from build123d import *

# Parameters (mm, degrees)
SKETCH_1_W          = 180
SKETCH_1_H          = 128
SKETCH_1_W_2        = 176
SKETCH_1_H_2        = 124
EXTRUDE_1_DEPTH     = 45
SKETCH_2_W          = 15
SKETCH_2_H          = 3
EXTRUDE_2_DEPTH     = 10
SKETCH_3_R          = 3
CUT_EXTRUDE_1_DEPTH = 10


with BuildPart() as part:
    # 草圖1 → 填料-伸長1 (new body)
    with BuildSketch(Plane.XY):
        Rectangle(SKETCH_1_W, SKETCH_1_H)
        Rectangle(SKETCH_1_W_2, SKETCH_1_H_2, mode=Mode.SUBTRACT)
    extrude(amount=EXTRUDE_1_DEPTH)

    # 草圖2 → 填料-伸長2 (add)
    with BuildSketch(Plane.XZ.offset(64)):
        with Locations((82.5, 43.5)):
            Rectangle(SKETCH_2_W, SKETCH_2_H)
        with Locations((-82.5, 43.5)):
            Rectangle(SKETCH_2_W, SKETCH_2_H)
    extrude_2 = extrude(amount=EXTRUDE_2_DEPTH)

    # 草圖3 → 除料-伸長1 (cut)
    with BuildSketch(Plane(origin=(0, 0, 42), x_dir=(-1, 0, 0), z_dir=(0, 0, -1))):
        with Locations((-82.5, -69)):
            Circle(SKETCH_3_R)
        with Locations((82.5, -69)):
            Circle(SKETCH_3_R)
    cut_extrude_1 = extrude(amount=-CUT_EXTRUDE_1_DEPTH, mode=Mode.SUBTRACT)

    # 鏡射1: 填料-伸長2 across plane
    add(extrude_2.mirror(Plane.ZX))

    # 鏡射3: 除料-伸長1 across plane
    add(cut_extrude_1.mirror(Plane.ZX), mode=Mode.SUBTRACT)


solid = part.part
Could you check a few things on this model? Use its own coordinates, in mm. A direction names the side the tool comes from. Give positions to 0.01 mm unless a question says otherwise; leave off trailing zeros. Order: outer loops, then holes, each group sorted by start corner. A loop starts at its lowest first (then second) coordinate and runs counter-clockwise, first axis right, second up. Notation, with made-up numbers: (83.5, 66.25) -> (110.5, 66.25) arc R26 cw to (110.5, 90.25) -> close; hole circle Ø11 at (12, 53). An arc over 180 degrees is marked (long way). Answer in a Markdown table with one row per item. Add a question column.
Item 1: For faces 4 (the flat face through (88, -1, 22)), 5 (the flat face through (86, -69, 42)), 6 (the flat face through (86, 69, 42)), 7 (the flat face through (80, -66, 45)), which set-ups out of +Z, -Z, +X, -X, +Y, -Y let a thin tool reach every point of the face, with its end or its side?
Item 2: We'd pull the mould along X, two halves only. Please class faces 1 (the flat face through (-79, -69, 42)), 2 (the flat face through (90, -1, 22)), 3 (the cylindrical face through (-80.1, -70.8, 43.5)): pulls with the +X half, pulls with the -X half, needs draft (parallel to the pull), parting line crosses it, or undercut.
Item 3: Imagine slicing it at C-C (z = 3.5). List the corners of the cut face in (x, y) for me.
Item 4: I'm going to push flat-ended pins straight in: P1, Ø22.5, axis at x = 39, z = 30.5, coming from the -Y side; P2, Ø22.5, axis at x = 1.5, z = 17.5, coming from the +Y side; P3, Ø3.5, axis at x = -82.5, y = 69, coming from the +Z side; P4, Ø8, axis at x = -80, y = -67, coming from the -Z side. Where does each tip first touch, or does it pass through?
Item 5: Imagine slicing it at B-B (y = 36). List the corners of the cut face in (x, z) for me, and give its area (3 significant figures).
Item 6: Imagine slicing it at D-D (y = -69). List the corners of the cut face in (x, z) for me.
Item 7: Please list where these lines run through material, in increasing order: probe 1 along Y at (x, z) = (-82.5, 42.85); probe 2 along X at (y, z) = (69, 44); probe 3 along X at (y, z) = (-26, 25.5).
Item 8: Imagine slicing it at A-A (x = -82.5). List the corners of the cut face in (y, z) for me.
Result:
| question | item | result |
|---|---|---|
| 1 | face 4 | +Z, -Z |
| 1 | face 5 | -Z, +X, -X, -Y |
| 1 | face 6 | -Z, +X, -X, +Y |
| 1 | face 7 | +Z, +X, -X, +Y, -Y |
| 2 | face 1 | needs draft |
| 2 | face 2 | pulls with the +X half |
| 2 | face 3 | undercut |
| 3 | outline | (-90, -64) -> (90, -64) -> (90, 64) -> (-90, 64) -> close; hole (-88, -62) -> (88, -62) -> (88, 62) -> (-88, 62) -> close |
| 4 | P1 | y = -64 |
| 4 | P2 | y = 64 |
| 4 | P3 | through |
| 4 | P4 | z = 0 |
| 5 | outline | (-90, 0) -> (-88, 0) -> (-88, 45) -> (-90, 45) -> close; (88, 0) -> (90, 0) -> (90, 45) -> (88, 45) -> close |
| 5 | area | 180 mm2 |
| 6 | outline | (-90, 42) -> (-85.5, 42) -> (-85.5, 45) -> (-90, 45) -> close; (-79.5, 42) -> (-75, 42) -> (-75, 45) -> (-79.5, 45) -> close; (75, 42) -> (79.5, 42) -> (79.5, 45) -> (75, 45) -> close; (85.5, 42) -> (90, 42) -> (90, 45) -> (85.5, 45) -> close |
| 7 | probe 1 | -74 to -72, -66 to -62, 62 to 66, 72 to 74 |
| 7 | probe 2 | -90 to -85.5, -79.5 to -75, 75 to 79.5, 85.5 to 90 |
| 7 | probe 3 | -90 to -88, 88 to 90 |
| 8 | outline | (-74, 42) -> (-72, 42) -> (-72, 45) -> (-74, 45) -> close; (-66, 42) -> (-64, 42) -> (-64, 0) -> (-62, 0) -> (-62, 45) -> (-66, 45) -> close; (62, 0) -> (64, 0) -> (64, 42) -> (66, 42) -> (66, 45) -> (62, 45) -> close; (72, 42) -> (74, 42) -> (74, 45) -> (72, 45) -> close |
